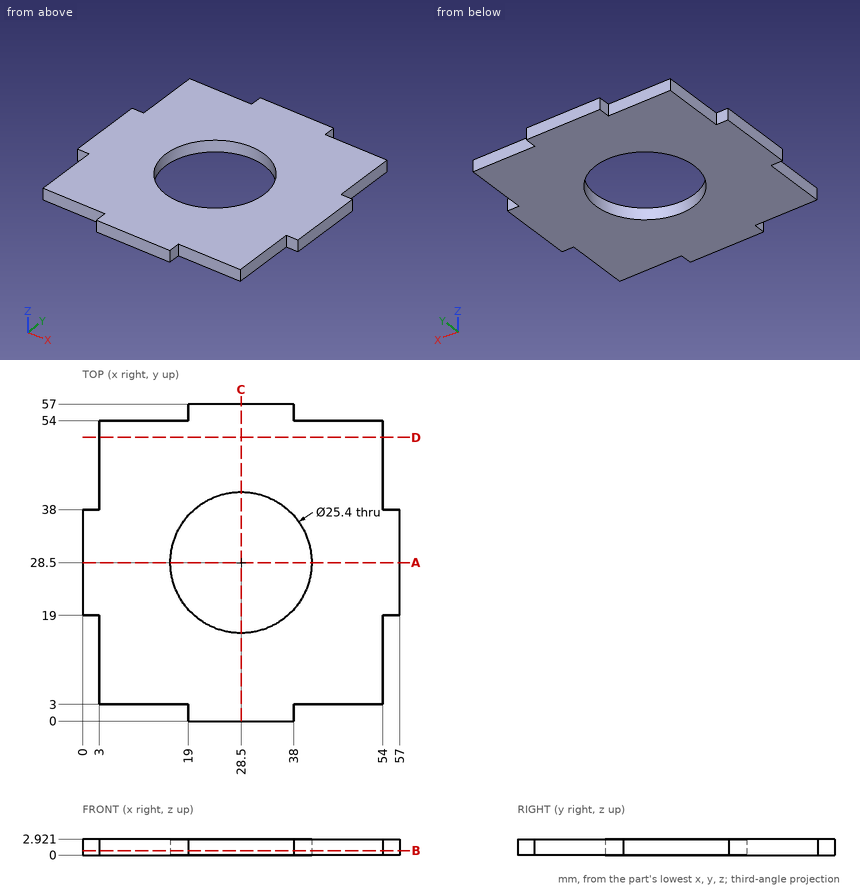
Study the drawing (mm; zero at the part's minimum x, y, z) and answer. Give positions to 0.01 mm unless a question says otherwise; leave off trailing zeros. Loops run counter-clockwise (first coordinate to the right, second up) from the corner with the lowest first, then second, coordinate; pieces in that order, holes last. Notation, with made-up numbers: (43, 18) - (76, 18) arc R20 cw to (76, 26) - close; hole circle Ø6 at (60.25, 46.5). An arc over 180 degrees is marked (long way). Answer as CSV lines item,"result". Start each with the question number.
1) Each of these flat-tipped pins is pushed along its axis until it touches: pin 1 Ø1.5 at (y, z) = (16, 2.5) entering from +X; pin 2 Ø1.5 at (x, z) = (12, 1) entering from +Y; pin 3 Ø0.9 at (y, z) = (1, 1.5) entering from -X. Where does it stop, or does it pass through?
2) Straight lines are drawn through the part: L1, parallel to Y at x = 28.5, z = 1.75; L2, parallel to X at y = 43, z = 2.65. For each, find the intervals that lie inside material, in ascending order. Write a range as from..to.
3) Find section B-B (z = 0.85). Write down the section's boundary in (x, y).
4) Find section A-A (y = 28.5). Write down the section's boundary in (x, z).
5) Find section D-D (y = 51). Write down the section's boundary in (x, z).
Findings below:
1,pin 1,"x = 54"
1,pin 2,"y = 54"
1,pin 3,"x = 19"
2,L1,"0..15.8, 41.2..57"
2,L2,"3..54"
3,outline,"(0, 19) - (3, 19) - (3, 3) - (19, 3) - (19, 0) - (38, 0) - (38, 3) - (54, 3) - (54, 19) - (57, 19) - (57, 38) - (54, 38) - (54, 54) - (38, 54) - (38, 57) - (19, 57) - (19, 54) - (3, 54) - (3, 38) - (0, 38) - close; hole circle Ø25.4 at (28.5, 28.5)"
4,outline,"(0, 0) - (15.8, 0) - (15.8, 2.92) - (0, 2.92) - close; (41.2, 0) - (57, 0) - (57, 2.92) - (41.2, 2.92) - close"
5,outline,"(3, 0) - (54, 0) - (54, 2.92) - (3, 2.92) - close"
